```python
from build123d import *

# Parameters (mm, degrees)
Y_KSEKLIK_EKSTR_ZYON1_DEPTH = 20
IZIM2_R                     = 12
KES_EKSTR_ZYON1_DEPTH       = 6
IZIM3_R                     = 6
KES_EKSTR_ZYON2_DEPTH       = 88.177978871
Y_KSEKLIK_EKSTR_ZYON2_DEPTH = 50
KES_EKSTR_ZYON3_DEPTH       = 111
KES_EKSTR_ZYON4_DEPTH       = 113.231902773
KES_EKSTR_ZYON5_DEPTH       = 113.231902773
KES_EKSTR_ZYON6_DEPTH       = 113.231902773


with BuildPart() as part:
    # Çizim1 → Yükseklik-Ekstrüzyon1 (new body)
    with BuildSketch(Plane.XY):
        with BuildLine():
            Line((40, -60), (-40, -60))
            ThreePointArc((-40, -60), (-54.142135624, -54.142135624), (-60, -40))
            Line((-60, -40), (-60, 40))
            ThreePointArc((-60, 40), (-54.142135624, 54.142135624), (-40, 60))
            Line((-40, 60), (40, 60))
            ThreePointArc((40, 60), (54.142135624, 54.142135624), (60, 40))
            Line((60, 40), (60, -40))
            ThreePointArc((60, -40), (54.142135624, -54.142135624), (40, -60))
        make_face()
    extrude(amount=Y_KSEKLIK_EKSTR_ZYON1_DEPTH)

    # Çizim2 → Kes-Ekstrüzyon1 (cut)
    with BuildSketch(Plane.XY.offset(20)):
        with Locations((-36, 36)):
            Circle(IZIM2_R)
        with Locations((36, 36)):
            Circle(IZIM2_R)
        with Locations((-36, -36)):
            Circle(IZIM2_R)
        with Locations((36, -36)):
            Circle(IZIM2_R)
    extrude(amount=-KES_EKSTR_ZYON1_DEPTH, mode=Mode.SUBTRACT)

    # Çizim3 → Kes-Ekstrüzyon2 (cut, through all)
    with BuildSketch(Plane.XY.offset(20)):
        with Locations((-36, 36)):
            Circle(IZIM3_R)
        with Locations((36, 36)):
            Circle(IZIM3_R)
        with Locations((36, -36)):
            Circle(IZIM3_R)
        with Locations((-36, -36)):
            Circle(IZIM3_R)
    extrude(amount=-KES_EKSTR_ZYON2_DEPTH, mode=Mode.SUBTRACT)

    # Çizim4 → Yükseklik-Ekstrüzyon2 (add)
    with BuildSketch(Plane.XY.offset(20)):
        with BuildLine():
            Line((4, -60), (-4, -60))
            Line((-4, -60), (-4, -29.732137495))
            ThreePointArc((-4, -29.732137495), (-21.213203436, -21.213203436), (-29.732137495, -4))
            Line((-29.732137495, -4), (-60, -4))
            Line((-60, -4), (-60, 4))
            Line((-60, 4), (-29.732137495, 4))
            ThreePointArc((-29.732137495, 4), (-21.213203436, 21.213203436), (-4, 29.732137495))
            Line((-4, 29.732137495), (-4, 60))
            Line((-4, 60), (4, 60))
            Line((4, 60), (4, 29.732137495))
            ThreePointArc((4, 29.732137495), (21.213203436, 21.213203436), (29.732137495, 4))
            Line((29.732137495, 4), (60, 4))
            Line((60, 4), (60, -4))
            Line((60, -4), (29.732137495, -4))
            ThreePointArc((29.732137495, -4), (21.213203436, -21.213203436), (4, -29.732137495))
            Line((4, -29.732137495), (4, -60))
        make_face()
    extrude(amount=Y_KSEKLIK_EKSTR_ZYON2_DEPTH)

    # Çizim5 → Kes-Ekstrüzyon3 (cut, through all)
    with BuildSketch(Plane.XY.offset(70)):
        with BuildLine():
            Line((7, 18.734993995), (7, 24))
            Line((7, 24), (-7, 24))
            Line((-7, 24), (-7, 18.734993995))
            ThreePointArc((-7, 18.734993995), (0, -20), (7, 18.734993995))
        make_face()
    extrude(amount=-KES_EKSTR_ZYON3_DEPTH, mode=Mode.SUBTRACT)

    # Çizim6 → Kes-Ekstrüzyon4 (cut, through all)
    with BuildSketch(Plane.ZY.offset(4)):
        Polygon((70, 60), (70, 29.732137495), (20, 60), align=None)
    extrude(amount=-KES_EKSTR_ZYON4_DEPTH, mode=Mode.SUBTRACT)

    # Çizim7 → Kes-Ekstrüzyon5 (cut, through all)
    with BuildSketch(Plane.ZY.offset(4)):
        Polygon((70, -29.732137495), (20, -60), (70, -60), align=None)
    extrude(amount=-KES_EKSTR_ZYON5_DEPTH, mode=Mode.SUBTRACT)

    # Çizim8 → Kes-Ekstrüzyon6 (cut, through all)
    with BuildSketch(Plane(origin=(0, 4, 0), x_dir=(1, 0, 0), z_dir=(0, 1, 0))):
        Polygon((-60, -20), (-29.732137495, -70), (-60, -70), align=None)
        Polygon((60, -20), (29.732137495, -70), (60, -70), align=None)
    extrude(amount=-KES_EKSTR_ZYON6_DEPTH, mode=Mode.SUBTRACT)


solid = part.part
```
Read the model definition and answer for the solid it produces. Units are mm, in the model's axes. A direction names the side the tool comes from. Round coordinates to 2 decimals unless told otherwise and drop trailing zeros. Write each loop counter-clockwise with the first axis right and the second up, starting at its lowest first coordinate (ties: lowest second). Pieces come first, ordered by that corner, then holes. Notation, with made-up numbers: (71.5, -29.5) -> (118.5, -29.5) arc R22 cw to (118.5, -3.5) -> close; hole circle Ø8 at (40.25, 88.5). An arc over 180 degrees is marked (long way). Answer in a Markdown table with one row per item. Add a question column.
1) Determine the mould class of faces 1 (the face through (21.019, 21.406, 44.65)), 2 (the face through (-21.406, 21.019, 44.65)), 3 (the face through (-42, 34, 14)) for opening direction X: pulls with the +X half, pulls with the -X half, needs draft (parallel to the pull), parting line crosses it, or undercut.
2) Find section D-D, the plane x = 33.5. Determine the outline of the cut face in (y, z), and give its area (3 significant figures).
3) Consider line 1 (Y direction, x = -36, z = 3.25); line 2 (Y direction, x = 36.5, z = 17.5); line 3 (X direction, y = 43, z = 15.5). Determine where each line is inside the solid, lowest interval first.
4) Find section B-B, the plane z = 48. Determine the outline of the cut face in (x, y) (3 decimals).
5) Given P1, Ø1.5, axis at x = -12, z = 45.5, coming from the -Y side; P2, Ø4, axis at y = 21, z = 38, coming from the -X side; P3, Ø8, axis at x = 31, y = -20, coming from the +Z side, each flat-ended and moving along its own axis, determine where each tip first touches the part or whether it passes through.
6) Find section A-A, the plane z = 11.5. Determine the outline of the cut face in (x, y) (3 decimals), and give its area (3 significant figures).
7) Which of the six approach directions +Z, -Z, +X, -X, +Y, -Y give full straight-line access (tool end or side, diameter ignored) to faces 4 (the face through (-7, 21, 35)), 5 (the face through (-42, -38, 14)), 6 (the face through (41, 4, 39)), 7 (the face through (21.406, -21.019, 44.65))?
8) Find section C-C, the plane y = -36. Determine the outline of the cut face in (x, z), and give its area (3 significant figures).
Findings below:
| question | item | result |
|---|---|---|
| 1 | face 1 | pulls with the +X half |
| 1 | face 2 | pulls with the -X half |
| 1 | face 3 | undercut |
| 2 | outline | (-60, 0) -> (-41.45, 0) -> (-41.45, 14) -> (-47.74, 14) -> (-47.74, 20) -> (-60, 20) -> close; (-30.55, 0) -> (30.55, 0) -> (30.55, 14) -> (24.26, 14) -> (24.26, 20) -> (4, 20) -> (4, 63.78) -> (-4, 63.78) -> (-4, 20) -> (-24.26, 20) -> (-24.26, 14) -> (-30.55, 14) -> close; (41.45, 0) -> (60, 0) -> (60, 20) -> (47.74, 20) -> (47.74, 14) -> (41.45, 14) -> close |
| 2 | area | 2,160 mm² |
| 3 | line 1 | -60 to -42, -30 to 30, 42 to 60 |
| 3 | line 2 | -60 to -47.99, -24.01 to 24.01, 47.99 to 60 |
| 3 | line 3 | -59.77 to -45.75, -26.25 to 26.25, 45.75 to 59.77 |
| 4 | outline | (-43.05, -4) -> (-29.732, -4) arc R30 ccw to (-4, -29.732) -> (-4, -43.05) -> (4, -43.05) -> (4, -29.732) arc R30 ccw to (29.732, -4) -> (43.05, -4) -> (43.05, 4) -> (29.732, 4) arc R30 ccw to (4, 29.732) -> (4, 43.05) -> (-4, 43.05) -> (-4, 29.732) arc R30 ccw to (-29.732, 4) -> (-43.05, 4) -> close; hole (-7, 18.735) arc R20 ccw (long way) to (7, 18.735) -> (7, 24) -> (-7, 24) -> close |
| 5 | P1 | y = -27.81 |
| 5 | P2 | x = -23.22 |
| 5 | P3 | z = 20 |
| 6 | outline | (-60, -40) arc R20 ccw to (-40, -60) -> (40, -60) arc R20 ccw to (60, -40) -> (60, 40) arc R20 ccw to (40, 60) -> (-40, 60) arc R20 ccw to (-60, 40) -> close; hole circle Ø12 at (-36, -36); hole circle Ø12 at (-36, 36); hole (-7, 18.735) arc R20 ccw (long way) to (7, 18.735) -> (7, 24) -> (-7, 24) -> close; hole circle Ø12 at (36, -36); hole circle Ø12 at (36, 36) |
| 6 | area | 12,300 mm² |
| 7 | face 4 | +Z, -Z |
| 7 | face 5 | +Z |
| 7 | face 6 | +Z, +X, +Y |
| 7 | face 7 | +Z, +X, -Y |
| 8 | outline | (-60, 0) -> (-42, 0) -> (-42, 14) -> (-48, 14) -> (-48, 20) -> (-60, 20) -> close; (-30, 0) -> (30, 0) -> (30, 14) -> (24, 14) -> (24, 20) -> (4, 20) -> (4, 59.65) -> (-4, 59.65) -> (-4, 20) -> (-24, 20) -> (-24, 14) -> (-30, 14) -> close; (42, 0) -> (60, 0) -> (60, 20) -> (48, 20) -> (48, 14) -> (42, 14) -> close |
| 8 | area | 2,090 mm² |
